Autodesk Fusion 360 part; units mm, degrees
sketch "Sketch1" plane through (0, 0, 0) normal (0, 0, 1) x (1, 0, 0)
  circle A0 centre (0, 0) radius 35.814
  circle A1 centre (0, 0) radius 38.1
  line L0 (-25, -25.6445) -> (25, -25.6445)
  line L1 (-25, 25.6445) -> (-25, -25.6445)
  line L2 (-25, 25.6445) -> (28.1774, 25.6445)
  line L3 (-25, 25.6445) -> (-28.1774, 25.6445)
  line L4 (-22, -31.1064) -> (-22, -28.2603)
  line L5 (-22, -28.2603) -> (22, -28.2603)
  line L6 (22, -31.1064) -> (22, -28.2603)
  line L7 (-25.1217, 28.6445) -> (25.1217, 28.6445)
  line L8 (12.5, 25.6445) -> (-12.5, 25.6445)
  line L9 (-12.5, 25.6445) -> (-12.5, 21.6445)
  line L10 (-12.5, 21.6445) -> (12.5, 21.6445)
  line L11 (12.5, 21.6445) -> (12.5, 25.6445)
  line L12 (14.5, 25.6445) -> (-14.5, 25.6445)
  line L13 (-14.5, 25.6445) -> (-14.5, 19.6445)
  line L14 (-14.5, 19.6445) -> (14.5, 19.6445)
  line L15 (14.5, 19.6445) -> (14.5, 25.6445)
  line L16 (0, 21.6445) -> (0, 25.6445)
  line L17 (0, 25.6445) -> (0, 0) construction
  line L18 (34.2402, 10.5) -> (29, 10.5)
  line L19 (29, 10.5) -> (29, -10.5)
  line L20 (29, -10.5) -> (34.2402, -10.5)
  line L21 (33.5618, -12.5) -> (27, -12.5)
  line L22 (27, -12.5) -> (27, 12.5)
  line L23 (27, 12.5) -> (33.5618, 12.5)
  line L24 (27, 0) -> (0, 0) construction
  line L25 (-27, -12.5) -> (-27, 12.5)
  line L26 (-29, 10.5) -> (-29, -10.5)
  line L27 (-34.2402, 10.5) -> (-29, 10.5)
  line L28 (-27, 12.5) -> (-33.5618, 12.5)
  line L29 (-29, -10.5) -> (-34.2402, -10.5)
  line L30 (-33.5618, -12.5) -> (-27, -12.5)
  dimension "d1" = 76.2
  dimension "d3" = 50
  dimension "d15" = 3
  dimension "d16" = 3
  dimension "d24" = 2
  dimension "d25" = 2
  dimension "d26" = 2
  dimension "d27" = 25
  dimension "d28" = 6
  dimension "d37" = 2
  dimension "d38" = 25
  dimension "d39" = 2
  dimension "d40" = 2
  dimension "d41" = 2
  dimension "d60" = 71.628
extrude "Extrude1" add sketch "Sketch1" along normal blind 55 contours A0 A1 L2 L6 | A0 L18 L19 L20 L21 L22 L23 | A0 L2 L7 L8 L12 | A0 A1 L2 L7 | A0 L0 L5 | A0 A1 L3 L4 | A0 A1 L3 L7 | A0 L25 L26 L27 L28 L29 L30
sketch "Sketch3" plane through (0, -25.6445, 0) normal (0, 1, 0) x (-1, 0, 0)
  line L0 (-25, 0) -> (25, 0)
  line L1 (25, 0) -> (25, 55)
  line L2 (25, 55) -> (-25, 55)
  line L3 (-25, 55) -> (-25, 0)
  line L4 (0, 0) -> (0, 27.5) construction
  line L5 (-25, 27.5) -> (0, 27.5) construction
  line L6 (0, 27.5) -> (-19.997, 7.503) construction
  circle A0 centre (-19.997, 7.503) radius 1.5
  circle A1 centre (-19.997, 7.503) radius 2.5
  circle A2 centre (19.997, 7.503) radius 2.5
  circle A3 centre (19.997, 7.503) radius 1.5
  circle A4 centre (19.997, 47.497) radius 2.5
  circle A5 centre (19.997, 47.497) radius 1.5
  circle A6 centre (-19.997, 47.497) radius 2.5
  circle A7 centre (-19.997, 47.497) radius 1.5
  dimension "d7" = 45
  dimension "d8" = 28.28
  dimension "d9" = 3
  dimension "d10" = 5
  dimension "d12" = 360
extrude "Extrude2" add sketch "Sketch3" along normal blind 25 contours A1 | A2 | A4 | A6
fillet "Fillet1" radius 2 2 edges at (22, -28.2603, 27.5) (-22, -28.2603, 27.5)
fillet "Fillet2" radius 5 4 edges at (25, -25.6445, 27.5) (25, -25.6445, 27.5) (25, 25.6445, 27.5) (25, 25.6445, 27.5)
extrude "Extrude3" cut sketch "Sketch1" along normal blind 15 contours A0 L18 L19 L20 L21 L22 L23 | L2 L9 L10 L11 L12 L13 L14 L15 | A0 L25 L26 L27 L28 L29 L30
sketch "Sketch5" plane through (0, 0, 55) normal (0, 0, 1) x (-1, 0, 0)
  arc A0 (34.2402, -10.5) -> (34.2402, 10.5) centre (0, 0) ccw
  line L0 (34.2402, -10.5) -> (29, -10.5)
  line L1 (29, -10.5) -> (29, 10.5)
  line L2 (29, 10.5) -> (34.2402, 10.5)
  line L3 (-22.8759, 25.6445) -> (25, 25.6445)
  arc A1 (33.5618, 12.5) -> (25, 25.6445) centre (0, 0) ccw
  line L4 (33.5618, 12.5) -> (27, 12.5)
  line L5 (27, 12.5) -> (27, -12.5)
  line L6 (27, -12.5) -> (33.5618, -12.5)
  arc A2 (25, -25.6445) -> (33.5618, -12.5) centre (0, 0) ccw
  line L7 (25, -25.6445) -> (-22.8759, -25.6445)
  arc A3 (-26.5878, -23.9944) -> (-22.8759, -25.6445) centre (-22.8759, -20.6445) ccw
  arc A4 (-33.5618, -12.5) -> (-26.5878, -23.9944) centre (0, 0) ccw
  line L8 (-33.5618, -12.5) -> (-27, -12.5)
  line L9 (-27, -12.5) -> (-27, 12.5)
  line L10 (-27, 12.5) -> (-33.5618, 12.5)
  arc A5 (-26.5878, 23.9944) -> (-33.5618, 12.5) centre (0, 0) ccw
  arc A6 (-22.8759, 25.6445) -> (-26.5878, 23.9944) centre (-22.8759, 20.6445) ccw
  line L11 (-34.2402, 10.5) -> (-29, 10.5)
  line L12 (-29, 10.5) -> (-29, -10.5)
  line L13 (-29, -10.5) -> (-34.2402, -10.5)
  arc A7 (-34.2402, 10.5) -> (-34.2402, -10.5) centre (0, 0) ccw
  line L14 (22, 31.1064) -> (22, 30.2603)
  arc A8 (20, 28.2603) -> (22, 30.2603) centre (20, 30.2603) ccw
  line L15 (20, 28.2603) -> (-20, 28.2603)
  arc A9 (-22, 30.2603) -> (-20, 28.2603) centre (-20, 30.2603) ccw
  line L16 (-22, 30.2603) -> (-22, 31.1064)
  arc A10 (-22, 31.1064) -> (-25.1217, -28.6445) centre (0, 0) ccw
  line L17 (-25.1217, -28.6445) -> (25.1217, -28.6445)
  arc A11 (25.1217, -28.6445) -> (22, 31.1064) centre (0, 0) ccw
  line L18 (-33.5618, -12.5) -> (-34.2402, -10.5)
  line L19 (-34.2402, 10.5) -> (-33.5618, 12.5)
  line L20 (34.2402, 10.5) -> (33.5618, 12.5)
  line L21 (34.2402, -10.5) -> (33.5618, -12.5)
extrude "Extrude5" cut sketch "Sketch5" against normal blind 15 contours L0 L1 L2 L4 L5 L6 L20 L21 | L8 L9 L10 L11 L12 L13 L18 L19
fillet "Fillet6" radius 5 1 edges at (-25, -25.6445, 27.5)
fillet "Fillet7" radius 1 15 edges at (27, 12.5, 27.5) (27, -12.5, 27.5) (33.5618, -12.5, 27.5) (34.2402, 10.5, 27.5) (33.5618, 12.5, 27.5) (-27, 12.5, 27.5) (-27, -12.5, 27.5) (-34.2402, -10.5, 27.5) (-29, -10.5, 27.5) (-29, 10.5, 27.5) (-33.5618, 12.5, 27.5) (-33.5618, -12.5, 27.5) (29, -10.5, 27.5) (29, 10.5, 27.5) (34.2402, -10.5, 27.5)
fillet "Fillet8" radius 1 1 edges at (-34.2402, 10.5, 27.5)
equation "d8 = 20 * 1.414 mm"
Work out the finished part from the listing and answer in its coordinate system (mm). A direction names the side the tool comes from. Round coordinates to 2 decimals unless told otherwise and drop trailing zeros. Loops run counter-clockwise (first coordinate to the right, second up) from the corner with the lowest first, then second, coordinate; pieces in that order, holes last. Notation, with made-up numbers: (5.25, 3) -> (34.25, 3) arc R11 cw to (34.25, 12) -> close; hole circle Ø9 at (39.5, 69.25). An arc over 180 degrees is marked (long way). Write each question's results on one line, items separated by ' | '. Start each with the question number.
1. Given pin 1 Ø1.7 at (x, z) = (31.5, 28.5) entering from +Y; pin 2 Ø3 at (y, z) = (2.5, 30.5) entering from +X; pin 3 Ø2.5 at (x, z) = (-19.997, 7.503) entering from -Y, each flat-ended and moving along its own axis, determine where each tip first touches the part or whether it passes through.
2. Find the intervals of material crossed by probe 1 along X at (y, z) = (-1, 36); probe 2 along X at (y, z) = (-18, 7.5); probe 3 along Y at (x, z) = (-9, 44), in increasing order. Write a range as from..to.
3. A tool of negligible diameter and unlimited length cuts with its end or side. For faces 1 (the face through (20, -25.644, 7)), 2 (the face through (33.9, 11.5, 47.6)), 3 (the face through (0, 28.644, 27)), 4 (the face through (-27, 0, 27)), from which of +Z, -Z, +X, -X, +Y, -Y can it reach the whole face along a straight path? Write none if from no direction.
4. For a pull along X with two mould halves and no side action, classify faces 5 (the face through (24.88, -25.225, 27.885)), 6 (the face through (3, -28, 55)) as +X half, -X half, draft (parallel to the pull), parting line (faces both ways), or undercut.
5. Section A-A (y = -23) is taken. State how many separate pieces and enclosed holes the cut face has, plus the area to 3 significant figures.
6. Section B-B (x = -8) is taken. Determine the outline of the cut face in (y, z).
Evaluation:
1) pin 1: stops at y = 22.63 | pin 2: stops at x = 38.09 | pin 3: stops at y = -28.7
2) probe 1: x = -38.09..-35.8, -29..-27, 27..29, 35.8..38.09 | probe 2: x = -33.58..-30.96, -22.5..-21.5, -18.5..-17.5, 17.5..18.5, 21.5..22.5, 30.96..33.58 | probe 3: y = -28.26..-25.64, 25.64..28.64
3) face 1: none | face 2: +Z | face 3: +Z, -Z, +X, -X, +Y | face 4: +Z, -Z
4) face 5: undercut | face 6: draft
5) separate pieces: 6 | enclosed holes: 4 | area: 372 mm2
6) outline: (-28.26, 0) -> (-25.64, 0) -> (-25.64, 55) -> (-28.26, 55) -> close; (25.64, 0) -> (28.64, 0) -> (28.64, 55) -> (25.64, 55) -> close
